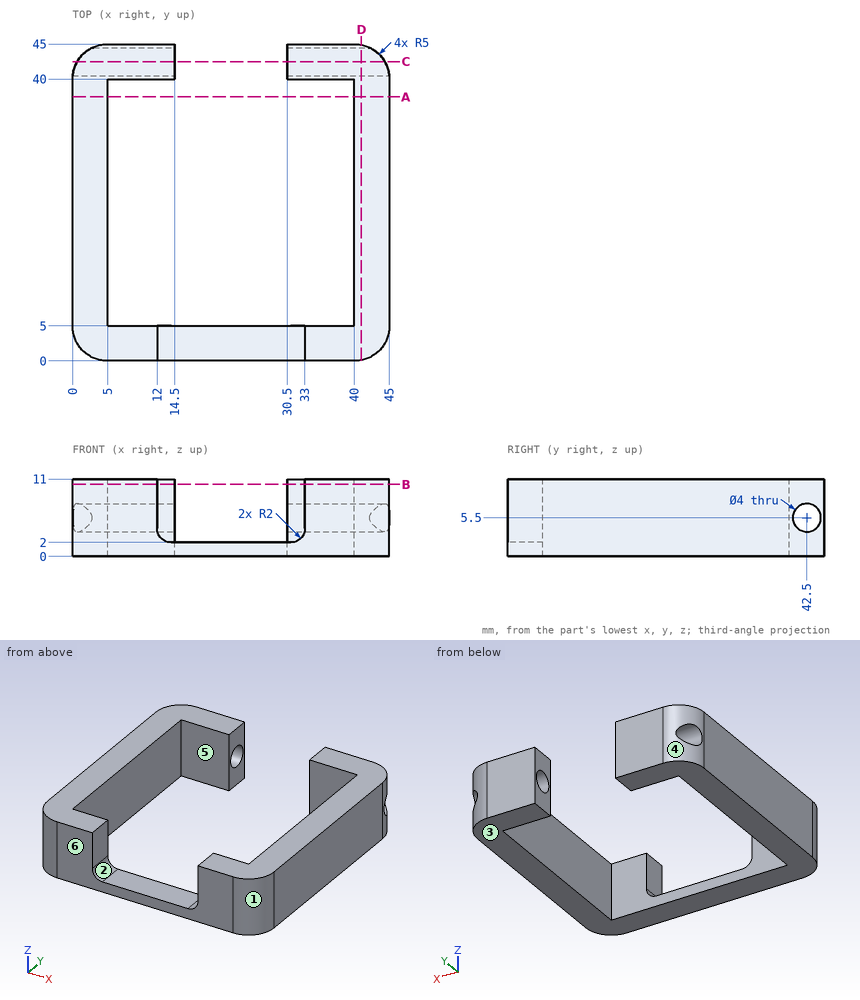
Geometry check sheet. Reference: drawing and pictorial views, mm from the part's lowest x, y, z. A direction names the side the tool comes from. Give positions to 0.01 mm unless a question says otherwise; leave off trailing zeros. Loops run counter-clockwise (first coordinate to the right, second up) from the corner with the lowest first, then second, coordinate; pieces in that order, holes last.
1. Go/stop test with flat-tipped pins: pin 1 Ø4 at (y, z) = (2, 7) entering from -X; pin 2 Ø1.5 at (y, z) = (42, 3) entering from -X; pin 3 Ø5.5 at (x, y) = (26.5, 1.5) entering from +Z; pin 4 Ø1.5 at (y, z) = (41.5, 6) entering from +X. Record where each tip stops, or that it passes through.
2. Section check C-C, the plane y = 42.5. Enter the section's corners in (x, z), then the cut area to 3 significant figures.
3. Section check D-D, the plane x = 41. Enter the section's corners in (y, z), then the cut area to 3 significant figures.
4. Section check A-A, the plane y = 37.5. Enter the section's corners in (x, z), then the cut area to 3 significant figures.
5. Thickness scan on line 1 (X direction, y = 23.5, z = 3.75); line 2 (Z direction, x = 8, y = 42.5). Record the ranges inside material, lowest first.
6. Section check B-B, the plane z = 10.25. Enter the section's corners in (x, y), then the cut area to 3 significant figures.
7. Set-up check for the marked faces 5 and 6: record each of +Z, -Z, +X, -X, +Y, -Y from which the full face is reachable in a straight line by a thin tool's end or side.
8. Mould release check, pull along X, two halves, no side actions. Record for the marked faces 1, 2, 3 and 4: released by +X, released by -X, zero draft, split by the parting line, or undercut.
Geometry says:
1. pin 1: stops at x = 0.1
1. pin 2: stops at x = 0.16
1. pin 3: stops at z = 2
1. pin 4: passes through
2. outline: (0.67, 0) - (14.5, 0) - (14.5, 3.5) - (0.67, 3.5) - close; (0.67, 7.5) - (14.5, 7.5) - (14.5, 11) - (0.67, 11) - close; (30.5, 0) - (44.33, 0) - (44.33, 3.5) - (30.5, 3.5) - close; (30.5, 7.5) - (44.33, 7.5) - (44.33, 11) - (30.5, 11) - close
2. area: 194 mm2
3. outline: (0.1, 0) - (44.9, 0) - (44.9, 11) - (0.1, 11) - close; hole circle Ø4 at (42.5, 5.5)
3. area: 480 mm2
4. outline: (0, 0) - (5, 0) - (5, 11) - (0, 11) - close; (40, 0) - (45, 0) - (45, 11) - (40, 11) - close
4. area: 110 mm2
5. line 1: x = 0 to 5, 40 to 45
5. line 2: z = 0 to 3.5, 7.5 to 11
6. outline: (0, 5) arc R5 ccw to (5, 0) - (12, 0) - (12, 5) - (5, 5) - (5, 40) - (14.5, 40) - (14.5, 45) - (5, 45) arc R5 ccw to (0, 40) - close; (30.5, 40) - (40, 40) - (40, 5) - (33, 5) - (33, 0) - (40, 0) arc R5 ccw to (45, 5) - (45, 40) arc R5 ccw to (40, 45) - (30.5, 45) - close
6. area: 594 mm2
7. face 5: +Z, -Z
7. face 6: +Z, -Z, +X, -X, -Y
8. face 1: released by +X
8. face 2: undercut
8. face 3: zero draft
8. face 4: released by -X
